Source: CAD feature listing. Evaluate the final solid. Frame: model axes, mm. A direction names the side the tool comes from. Give positions to 0.01 mm unless a question says otherwise; leave off trailing zeros. Loops run counter-clockwise (first coordinate to the right, second up) from the corner with the lowest first, then second, coordinate; pieces in that order, holes last. Notation, with made-up numbers: (84, 75.5) -> (110, 75.5) arc R24 cw to (110, 96.5) -> close; hole circle Ø4 at (83.25, -37.5). An arc over 180 degrees is marked (long way). Put each result on its own line as item: value.
```python
from build123d import *

# Parameters (mm, degrees)
ESQUISSE1_W                             = 250
ESQUISSE1_H                             = 100
BOSS_EXTRU_1_DEPTH                      = 10
ESQUISSE2_OUTSIDE_W                     = 305.888
ESQUISSE2_OUTSIDE_H                     = 155.888
ENL_V_MAT_EXTRU_1_DEPTH                 = 270.443871706
ENL_V_MAT_EXTRU_2_DEPTH                 = 270.443871706
CONG_1_R                                = 15
ESQUISSE4_R                             = 3.305
ENL_V_MAT_EXTRU_3_DEPTH                 = 270.443640324
PER_AGE_POUR_CROUS_AUTO_BLOQUANTS_300_D = 4.7625
PER_AGE_POUR_CROUS_AUTO_BLOQUANTS_3_2_D = 4.7625
ENL_V_MAT_EXTRU_4_DEPTH                 = 10


with BuildPart() as part:
    # Esquisse1 → Boss.-Extru.1 (new body)
    with BuildSketch(Plane.XY):
        with Locations((125, 50)):
            Rectangle(ESQUISSE1_W, ESQUISSE1_H)
    extrude(amount=BOSS_EXTRU_1_DEPTH)

    # Esquisse2 outside → Enlèv. mat.-Extru.1 (cut, through all)
    with BuildSketch(Plane.XY.offset(10)):
        with Locations((125, 50)):
            Rectangle(ESQUISSE2_OUTSIDE_W, ESQUISSE2_OUTSIDE_H)
        Polygon((250, 83.248936833), (155, 100), (45, 90.376247012), (0, 73.99758647), (0, 23.99758647), (41.565039025, 0), (126.565039025, 0), (145.081949739, 8.634577271), (165.081949739, 43.275593423), (250, 58.248936833), align=None, mode=Mode.SUBTRACT)
    extrude(amount=-ENL_V_MAT_EXTRU_1_DEPTH, mode=Mode.SUBTRACT)

    # Esquisse3 → Enlèv. mat.-Extru.2 (cut, through all)
    with BuildSketch(Plane.XY.offset(10)):
        Polygon((134.456309599, 20.230428685), (155.141265019, 56.057822426), (132.800938883, 83.000536248), (68.90430085, 77.410304783), (121.374682449, 14.130365764), align=None)
        Polygon((105.313706387, 10), (74.046358719, 47.708813875), (60.975248723, 36.870527049), align=None)
        Polygon((20, 26.375291272), (20, 37.889147432), (40, 37.889147432), (86.019260451, 10), (28.660254038, 21.375291272), align=None)
        Polygon((20, 61.702841638), (48.147118965, 44.644785014), (65, 58.618836074), (49.418513209, 77.410304783), (20, 66.702841638), align=None)
    extrude(amount=-ENL_V_MAT_EXTRU_2_DEPTH, mode=Mode.SUBTRACT)

    # Congé1
    # the kernel refuses this fillet: 15 mm, written as the material it takes off along each edge
    with BuildSketch(Plane(origin=(250, 83.248936833, 41.466236169), x_dir=(-0.9848077530122094, 0.17364817766692334, 0), z_dir=(0, 0, -1))) as cong_1_piece_1:
        with BuildLine():
            CenterArc((CONG_1_R * 0.839099631177, -CONG_1_R), CONG_1_R, 90, 80)
            Line((-CONG_1_R * 0.145708121835, -CONG_1_R * 0.826351822333), (0, 0))
            Line((0, 0), (CONG_1_R * 0.839099631177, 0))
        make_face()
    extrude(amount=72.932472338, mode=Mode.SUBTRACT)
    with BuildSketch(Plane(origin=(250, 58.248936833, 41.466236169), x_dir=(-0.984807753012208, -0.17364817766693091, 0), z_dir=(0, 0, -1))) as cong_1_piece_2:
        with BuildLine():
            CenterArc((CONG_1_R * 0.839099631177, CONG_1_R), CONG_1_R, 190, 80)
            Line((-CONG_1_R * 0.145708121835, CONG_1_R * 0.826351822333), (0, 0))
            Line((0, 0), (CONG_1_R * 0.839099631177, 0))
        make_face()
    extrude(amount=72.932472338, mode=Mode.SUBTRACT)

    # Esquisse4 → Enlèv. mat.-Extru.3 (cut, through all)
    with BuildSketch(Plane.XY.offset(10)):
        with Locations((224.999750621, 60.537155323)):
            Circle(ESQUISSE4_R)
    extrude(amount=-ENL_V_MAT_EXTRU_3_DEPTH, mode=Mode.SUBTRACT)

    # Per_age pour _crous auto-bloquants 300 (through all)
    with Locations(Plane.XY.offset(10)):
        with Locations((85.764023291, 45.327215553), (143.900469441, 91.500268124)):
            Hole(PER_AGE_POUR_CROUS_AUTO_BLOQUANTS_300_D / 2)

    # Per_age pour _crous auto-bloquants 3 2 (through all)
    with Locations(Plane.XY.offset(10)):
        with Locations((10, 64.202841638), (10, 33.792331302)):
            Hole(PER_AGE_POUR_CROUS_AUTO_BLOQUANTS_3_2_D / 2)

    # Esquisse10 → Enlèv. mat.-Extru.4 (cut)
    with BuildSketch(Plane.XY.offset(10)):
        Polygon((174.373076709, 89.029229885), (173.279093189, 82.824941041), (193.270690575, 79.299883034), (194.364674095, 85.504171878), align=None)
    extrude(amount=-ENL_V_MAT_EXTRU_4_DEPTH, mode=Mode.SUBTRACT)


solid = part.part
```
(1) Line query: probe 1 along Y at (x, z) = (10, 5); probe 2 along Y at (x, z) = (66, 7.75); probe 3 along X at (y, z) = (24, 4.5). Output: solid intervals per line, ascending. Write a range as from..to.
Calculated:
probe 1: y = 18.22..31.41, 36.17..61.82, 66.58..77.64
probe 2: y = 0..13.97, 22.13..33.83, 41.04..92.21
probe 3: x = 0..24.11, 62.92..82.21, 93.71..113.19, 136.63..153.95
(2) Section A-A on x = 10. Return loops of the section in (y, z), then the cut area to 3 significant figures.
Calculated:
outline: (18.22, 0) -> (31.41, 0) -> (31.41, 10) -> (18.22, 10) -> close; (36.17, 0) -> (61.82, 0) -> (61.82, 10) -> (36.17, 10) -> close; (66.58, 0) -> (77.64, 0) -> (77.64, 10) -> (66.58, 10) -> close
area: 499 mm²
(3) Draft query along X for faces 3 (the flat face through (33.88, 53.29, 5.07)), 4 (the flat face through (154.94, 25.71, 5.07)), 5 (the flat face through (20.492, 12.167, 5.07)), 6 (the flat face through (95, 40, 0)). Return one class per face: released by +X, released by -X, zero draft, split by the parting line, or undercut.
Calculated:
face 3: undercut
face 4: released by +X
face 5: released by -X
face 6: zero draft
(4) Section B-B on z = 5.5. Give the number of separate pieces and of enclosed holes in the cut face, then the cut area to 3 significant figures.
Calculated:
separate pieces: 1
enclosed holes: 10
area: 11,900 mm²
(5) Reachability of faces 1 (the flat face through (183.135, 81.087, 5.07)), 2 (the flat face through (196.881, 92.615, 5.07)) from +Z, -Z, +X, -X, +Y, -Y: full face, straight path, thin tool, end or side. Return the list, or none.
Calculated:
face 1: +Z, -Z
face 2: +Z, -Z, +X, +Y
(6) First-contact query: P1, Ø10.5, axis at x = 225, y = 60.54, coming from the -Z side; P2, Ø3, axis at x = 29.5, z = 7.5, coming from the -Y side; P3, Ø4, axis at x = 10, y = 64.2, coming from the +Z side; P4, Ø5, axis at x = 196, z = 4, coming from the +Y side. Flat tips, straight axial feed; report the tip coordinate or a pass-through.
Calculated:
P1: stops at z = 0
P2: stops at y = 6.1
P3: passes through
P4: stops at y = 93.21
